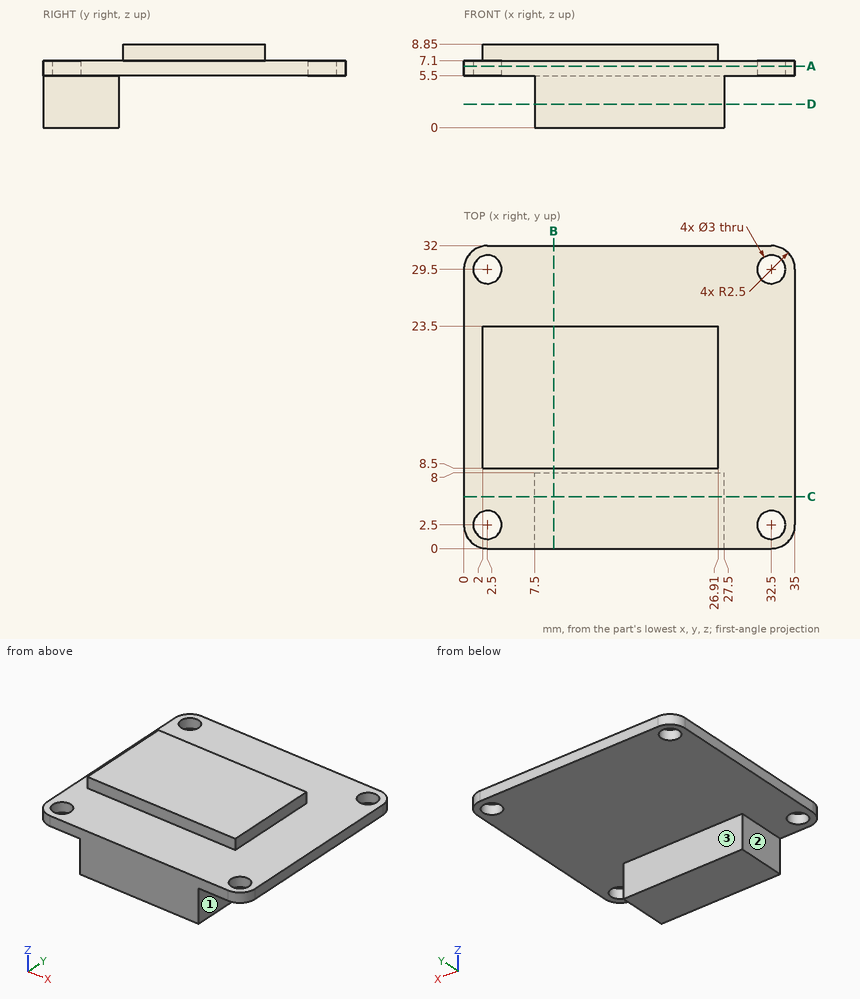
Answer from the drawing. Dimensions are ordinates in mm from the lowest x, y and z of the part. A direction names the side the tool comes from. Coordinates: 2 decimals unless noted, no trailing zeros. Order: outer loops, then holes, each group sorted by start corner. A loop starts at its lowest first (then second) coordinate and runs counter-clockwise, first axis right, second up. Notation, with made-up numbers: (16, 70.5) - (41, 70.5) arc R28 ccw to (41, 93.5) - close; hole circle Ø2 at (85, 34.5). An arc over 180 degrees is marked (long way). Answer as a JSON object with one key per item and string values. Group by question number.
Item 1: Section C-C (y = 5.5) is taken. Give the vertices of the cut face in (x, z).
Item 2: Section B-B (x = 9.5) is taken. Give the vertices of the cut face in (y, z).
Item 3: A tool of negligible diameter and unlimited length cuts with its end or side. For the marked faces 1, 2 and 3, from which of +Z, -Z, +X, -X, +Y, -Y can it reach the whole face along a straight path? Write none if from no direction.
Item 4: Section D-D (z = 2.5) is taken. Give the vertices of the cut face in (x, y).
Item 5: Flat-ended cylindrical pins translate along their axes: P1, Ø0.5, axis at x = 18.5, z = 8, coming from the -Y side; P2, Ø9.5, axis at x = 24.5, y = 13, coming from the -Z side; P3, Ø1.4, axis at y = 16, z = 8, coming from the -X side. Find the tip coordinate at first contact, or state that the pin passes through.
Item 6: Section A-A (z = 6.5) is taken. Give the vertices of the cut face in (x, y).
Item 7: Consider probe 1 along Z at (x, y) = (19, 2); probe 2 along Z at (x, y) = (21, 9); probe 3 along X at (y, z) = (11, 7.25). Determine where each line is inside the solid, lowest interval first. Write a range as from..to.
Results are:
{
 "1": {"outline": "(0, 5.5) - (7.5, 5.5) - (7.5, 0) - (27.5, 0) - (27.5, 5.5) - (35, 5.5) - (35, 7.1) - (0, 7.1) - close"},
 "2": {"outline": "(0, 0) - (8, 0) - (8, 5.5) - (32, 5.5) - (32, 7.1) - (23.5, 7.1) - (23.5, 8.85) - (8.5, 8.85) - (8.5, 7.1) - (0, 7.1) - close"},
 "3": {"face 1": "-Z, +X, +Y, -Y", "face 2": "-Z, -X, +Y, -Y", "face 3": "-Z, +X, -X, +Y"},
 "4": {"outline": "(7.5, 0) - (27.5, 0) - (27.5, 8) - (7.5, 8) - close"},
 "5": {"P1": "stops at y = 8.5", "P2": "stops at z = 5.5", "P3": "stops at x = 2"},
 "6": {"outline": "(0, 2.5) arc R2.5 ccw to (2.5, 0) - (32.5, 0) arc R2.5 ccw to (35, 2.5) - (35, 29.5) arc R2.5 ccw to (32.5, 32) - (2.5, 32) arc R2.5 ccw to (0, 29.5) - close; hole circle Ø3 at (2.5, 2.5); hole circle Ø3 at (2.5, 29.5); hole circle Ø3 at (32.5, 2.5); hole circle Ø3 at (32.5, 29.5)"},
 "7": {"probe 1": "z = 0..7.1", "probe 2": "z = 5.5..8.85", "probe 3": "x = 2..26.91"}
}
